Geometry check sheet. Reference: the model listing, model coordinates, mm. Face numbers are marked on the shaded views. Coordinates: 2 decimals unless noted, no trailing zeros. Order: outer loops, then holes, each group sorted by start corner. A loop starts at its lowest first (then second) coordinate and runs counter-clockwise, first axis right, second up.
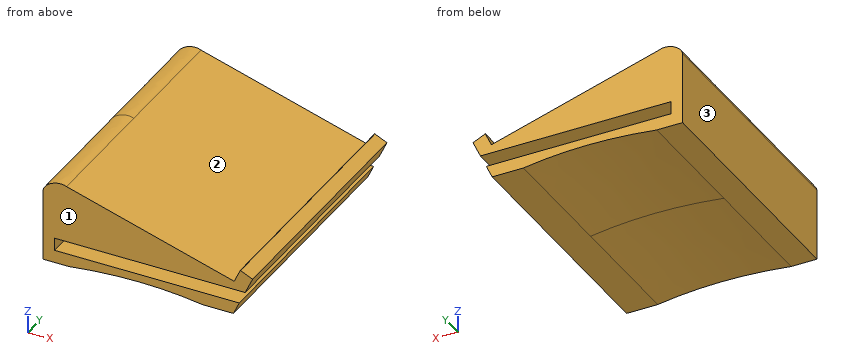
```python
from build123d import *

# Parameters (mm, degrees)
F0_W     = 16.392636
F0_H     = 18
F1_DEPTH = 179.45


with BuildPart() as f1:
    # F0 (on Front) → F1 (new body, symmetric)
    with BuildSketch(Plane.XZ):
        with BuildLine():
            Line((-125.372112, 36), (144.191556, 36))
            Line((144.191556, 36), (154.716455, 58.825539))
            Line((154.716455, 58.825539), (137.690631, 66.589023))
            Line((137.690631, 66.589023), (137.873941, 66.991033))
            Line((137.873941, 66.991033), (137.500362, 67.161379))
            Line((137.500362, 67.161379), (128.665014, 48))
            Line((128.665014, 48), (-108.450002, 117.533296))
            add(Edge.make_bspline(
                [(-141.764748, 102.030654), (-140.029642, 114.253703), (-119.663181, 122.909447), (-108.450002, 117.533296)],
                knots=[0, 0, 0, 0, 36.745125, 36.745125, 36.745125, 36.745125], degree=3))
            Line((-141.764748, 102.030654), (-141.764748, 36))
            Line((-141.764748, 36), (-125.372112, 36))
        make_face()
        with BuildLine():
            add(Edge.make_bspline(
                [(-105.076713, 0), (-42.760202, 8.42147), (21.213201, 9.788831), (83.456889, 0)],
                knots=[0, 0, 0, 0, 188.533601, 188.533601, 188.533601, 188.533601], degree=3))
            Line((83.456889, 0), (127.591888, 0))
            Line((127.591888, 0), (135.891722, 18))
            Line((135.891722, 18), (-125.372112, 18))
            Line((-125.372112, 18), (-141.764748, 18))
            Line((-141.764748, 18), (-141.764748, 0))
            Line((-141.764748, 0), (-105.076713, 0))
        make_face()
        with Locations((-133.56843, 27)):
            Rectangle(F0_W, F0_H)
    extrude(amount=F1_DEPTH, both=True)


solid = f1.part
```
Item 1: Depth check by flat-ended pin: P1, Ø20, axis at y = 62.5, z = 27.5, coming from the +X side; P2, Ø5, axis at x = 75, y = -85.5, coming from the -Z side; P3, Ø12, axis at x = 82, y = -61, coming from the +Z side. Enter the tip coordinate at first touch or a pass-through.
Item 2: Thickness scan on line 1 along Z through (x, y) = (99.5, 108); line 2 along Z through (x, y) = (116, 120); line 3 along X through (y, z) = (140, 11.5). Record the ranges inside material, lowest first.
Item 3: Release check for a two-part mould opening along X. For the marked faces 1, 2 and 3 record: pulls with the +X half, pulls with the -X half, needs draft (parallel to the pull), parting line crosses it, or undercut.
Item 4: Sectioned sample at A-A (z = 87). Record the cut outline in (x, y).
Geometry check:
1. P1: stops at x = 144.88
1. P2: stops at z = 0.9
1. P3: stops at z = 63.44
2. line 1: z = 0 to 18, 36 to 56.55
2. line 2: z = 0 to 18, 36 to 51.71
2. line 3: x = -141.76 to 132.89
3. face 1: needs draft
3. face 2: undercut
3. face 3: pulls with the -X half
4. outline: (-141.76, -179.45) - (-4.33, -179.45) - (-4.33, 179.45) - (-141.76, 179.45) - close
